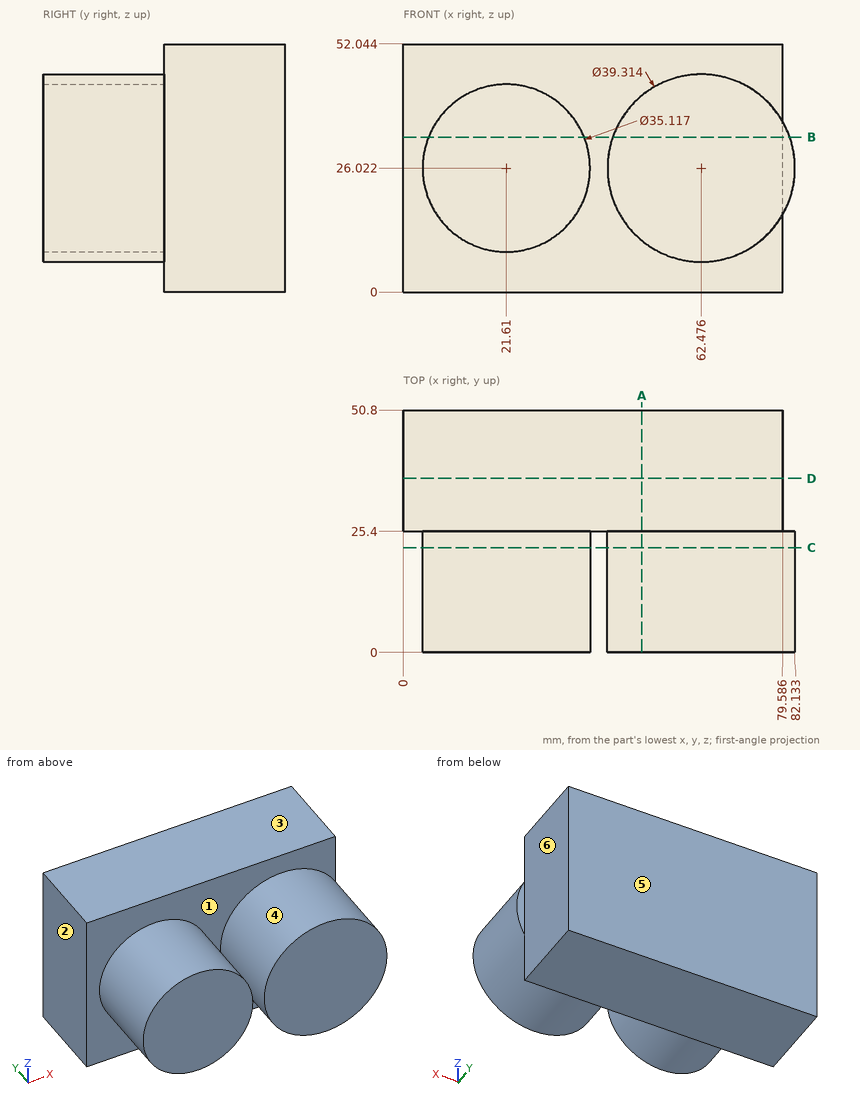
The figure shows three views and two pictorial views of one solid part (mm, origin at its lowest corner). Answer the questions. A direction names the side the tool comes from. Round coordinates to 2 decimals unless told otherwise and drop trailing zeros. Order: outer loops, then holes, each group sorted by start corner. A loop starts at its lowest first (then second) coordinate and runs counter-clockwise, first axis right, second up. Notation, with made-up numbers: (58, 29) - (117, 29) arc R7 ccw to (117, 37) - close; hole circle Ø8 at (-18, 57). An arc over 180 degrees is marked (long way). Write item = value, one per line. Start each with the question number.
1) For a pull along X with two mould halves and no side action, classify the marked faces 1, 2 and 3 as released by +X, released by -X, zero draft, split by the parting line, or undercut.
2) Given pin 1 (6 mm diameter, centred on y = 18, z = 22, fed in from -X); pin 2 (7.5 mm diameter, centred on y = 34.5, z = 22, fed in from +X); pin 3 (1 mm diameter, centred on y = 21, z = 39.5, fed in from -X) (1 decimal), each flat-ended and moving along its own axis, determine where each tip first touches the part or whether it passes through.
3) Section D-D, the plane y = 36.5 is taken. Write down the section's boundary in (x, z), plus the area to 3 significant figures.
4) Section B-B, the plane z = 32.5 is taken. Write down the section's boundary in (x, y) (1 decimal), plus the area to 3 significant figures.
5) Section C-C, the plane y = 22 is taken. Write down the section's boundary in (x, z) (1 decimal).
6) For the marked faces 4, 5 and 6, determine the directions among +Z, -Z, +X, -X, +Y, -Y from which every point of the face is accessible in a straight line to the end or side of a thin tool.
7) Section A-A, the plane x = 50 is taken. Write down the section's boundary in (y, z).
8) Straight lines are drawn through the part: L1, parallel to X at y = 34, z = 42; L2, parallel to Y at x = 45, z = 39.5; L3, parallel to X at y = 8.5, z = 28.5 (1 decimal). For each, find the intervals that lie inside material, in ascending order.
Results list:
q1.face_1 = undercut
q1.face_2 = released by -X
q1.face_3 = zero draft
q2.pin_1 = 4.08
q2.pin_2 = 79.59
q2.pin_3 = 9.8
q3.outline = (0, 0) - (79.59, 0) - (79.59, 52.04) - (0, 52.04) - close
q3.area = 4,140 mm^2
q4.outline = (0, 25.4) - (5.3, 25.4) - (5.3, 0) - (37.9, 0) - (37.9, 25.4) - (43.9, 25.4) - (43.9, 0) - (81, 0) - (81, 25.4) - (79.6, 25.4) - (79.6, 50.8) - (0, 50.8) - close
q4.area = 3,790 mm^2
q5.outline = circle Ø35.1 at (21.6, 26); circle Ø39.3 at (62.5, 26)
q6.face_4 = -Y
q6.face_5 = +Z, -Z, +X, -X, +Y
q6.face_6 = +Z, -Z, +X, +Y
q7.outline = (0, 10.83) - (25.4, 10.83) - (25.4, 0) - (50.8, 0) - (50.8, 52.04) - (25.4, 52.04) - (25.4, 41.21) - (0, 41.21) - close
q8.L1 = 0 to 79.59
q8.L2 = 25.4 to 50.8
q8.L3 = 4.2 to 39, 43 to 82
